from build123d import *

# Parameters (mm, degrees)
SKETCH1_R                             = 30
SKETCH1_R_2                           = 20
BOSS_EXTRUDE1_DEPTH                   = 40
TAP_DRILL_FOR_M8X1_25_TAP1_AT_2_COUNT = 2
TAP_DRILL_FOR_M8X1_25_TAP1_AT_2_PITCH = 40
TAP_DRILL_FOR_M8X1_25_TAP1_AT_3_COUNT = 2
TAP_DRILL_FOR_M8X1_25_TAP1_AT_3_PITCH = 50
TAP_DRILL_FOR_M8X1_25_TAP1_AT_4_COUNT = 2
TAP_DRILL_FOR_M8X1_25_TAP1_AT_4_PITCH = 30


with BuildPart() as part:
    # Sketch1 → Boss-Extrude1 (new, symmetric)
    with BuildSketch(Plane.XY):
        Circle(SKETCH1_R)
        Circle(SKETCH1_R_2, mode=Mode.SUBTRACT)
    extrude(amount=BOSS_EXTRUDE1_DEPTH, both=True)

    # Sketch12 → Tap Drill for M8x1.25 Tap1 (revolve, cut)
    with BuildSketch(Plane(origin=(-20, 15, 40), x_dir=(0, -1, 0), z_dir=(1, 0, 0))):
        Polygon((0, 0), (0, 22.042926105), (3.4, 20), (3.4, 0), align=None)
    tap_drill_for_m8x1_25_tap1 = revolve(axis=Axis((-20, 15, 46.35), (0, 0, -1)), mode=Mode.SUBTRACT)

    # Tap Drill for M8x1.25 Tap1 at 2: Tap Drill for M8x1.25 Tap1 ×2
    with Locations(*[(i * TAP_DRILL_FOR_M8X1_25_TAP1_AT_2_PITCH, 0, 0) for i in range(1, TAP_DRILL_FOR_M8X1_25_TAP1_AT_2_COUNT)]):
        add(tap_drill_for_m8x1_25_tap1, mode=Mode.SUBTRACT)

    # Tap Drill for M8x1.25 Tap1 at 3: Tap Drill for M8x1.25 Tap1 ×2
    with Locations(*[Vector(0.7999999999999999, -0.6000000000000001, 0) * (i * TAP_DRILL_FOR_M8X1_25_TAP1_AT_3_PITCH) for i in range(1, TAP_DRILL_FOR_M8X1_25_TAP1_AT_3_COUNT)]):
        add(tap_drill_for_m8x1_25_tap1, mode=Mode.SUBTRACT)

    # Tap Drill for M8x1.25 Tap1 at 4: Tap Drill for M8x1.25 Tap1 ×2
    with Locations(*[(0, -i * TAP_DRILL_FOR_M8X1_25_TAP1_AT_4_PITCH, 0) for i in range(1, TAP_DRILL_FOR_M8X1_25_TAP1_AT_4_COUNT)]):
        add(tap_drill_for_m8x1_25_tap1, mode=Mode.SUBTRACT)

    # Mirror1: Tap Drill for M8x1.25 Tap1 across plane
    add(tap_drill_for_m8x1_25_tap1.mirror(Plane.XY), mode=Mode.SUBTRACT)

    # Mirror1 copy 1 sketch → Mirror1 copy 1 (revolve, cut)
    with BuildSketch(Plane(origin=(20, 15, -40), x_dir=(0, -1, 0), z_dir=(1, 0, 0))):
        Polygon((0, 0), (0, -22.042926105), (3.4, -20), (3.4, 0), align=None)
    revolve(axis=Axis((20, 15, -46.35), (0, 0, -1)), mode=Mode.SUBTRACT)

    # Mirror1 copy 2 sketch → Mirror1 copy 2 (revolve, cut)
    with BuildSketch(Plane(origin=(20, -15, -40), x_dir=(0, -1, 0), z_dir=(1, 0, 0))):
        Polygon((0, 0), (0, -22.042926105), (3.4, -20), (3.4, 0), align=None)
    revolve(axis=Axis((20, -15, -46.35), (0, 0, -1)), mode=Mode.SUBTRACT)

    # Mirror1 copy 3 sketch → Mirror1 copy 3 (revolve, cut)
    with BuildSketch(Plane(origin=(-20, -15, -40), x_dir=(0, -1, 0), z_dir=(1, 0, 0))):
        Polygon((0, 0), (0, -22.042926105), (3.4, -20), (3.4, 0), align=None)
    revolve(axis=Axis((-20, -15, -46.35), (0, 0, -1)), mode=Mode.SUBTRACT)


solid = part.part
Model file for the job. Use its own axes, mm. A direction names the side the tool comes from. Round coordinates to 2 decimals unless told otherwise and drop trailing zeros. Loops run counter-clockwise (first coordinate to the right, second up) from the corner with the lowest first, then second, coordinate; pieces in that order, holes last. Notation, with made-up numbers: (7, -19.75) -> (37, -19.75) arc R22 ccw to (37, -12.75) -> close; hole circle Ø4 at (7, 18). An arc over 180 degrees is marked (long way). Answer as CSV lines item,"result". Start each with the question number.
1) Slice it at B-B (y = -6). List the corners of the cut face in (x, z).
2) Tool access for faces 1 (the face through (23.32, -14.26, -30.14)), 2 (the face through (-16.68, -14.26, 30.14)): list every direction of +Z, -Z, +X, -X, +Y, -Y with a clear straight run to the whole face (end or side of a thin tool).
3) Slice it at D-D (z = 2). List the corners of the cut face in (x, y).
4) Slice it at A-A (x = 0). List the corners of the cut face in (y, z), plus the area to 3 significant figures.
5) Mould opens along Y. For faces 3 (the face through (-4.336, -19.524, -0.56)), 4 (the face through (20, -6, 40)), 5 (the face through (-29.97, 1.32, 0.56)), 6 (the face through (-16.68, 15.74, -30.14)) say: +Y half, -Y half, draft (parallel to the pull), parting line (faces both ways), or undercut.
6) Slice it at C-C (z = -32). List the corners of the cut face in (x, y), plus the area to 3 significant figures.
7) Pin check, flat tips, straight feed: P1, Ø1, axis at y = -16, z = 4.5, coming from the -X side; P2, Ø8, axis at x = -12.5, z = 15.5, coming from the -Y side; P3, Ø8, axis at x = -12.5, z = -16, coming from the +Y side. Stop position of each tip, or through.
8) Probe line 1 along X through (y, z) = (-15, 29); line 2 along X through (y, z) = (-16, 20.5); line 3 along Y through (x, z) = (-5, -31.5). List the from-to ranges inside material, lowest first.
Filled in:
1,outline,"(-29.39, -40) -> (-19.08, -40) -> (-19.08, 40) -> (-29.39, 40) -> close; (19.08, -40) -> (29.39, -40) -> (29.39, 40) -> (19.08, 40) -> close"
2,face 1,"-Z"
2,face 2,"+Z"
3,outline,"circle Ø60 at (0, 0); hole circle Ø40 at (0, 0)"
4,outline,"(-30, -40) -> (-20, -40) -> (-20, 40) -> (-30, 40) -> close; (20, -40) -> (30, -40) -> (30, 40) -> (20, 40) -> close"
4,area,"1,600 mm2"
5,face 3,"undercut"
5,face 4,"draft"
5,face 5,"parting line"
5,face 6,"undercut"
6,outline,"circle Ø60 at (0, 0); hole circle Ø6.8 at (-20, -15); hole circle Ø6.8 at (-20, 15); hole circle Ø40 at (0, 0); hole circle Ø6.8 at (20, -15); hole circle Ø6.8 at (20, 15)"
6,area,"1,430 mm2"
7,P1,"stops at x = -25.69"
7,P2,"stops at y = -28.77"
7,P3,"stops at y = 28.77"
8,line 1,"x = -25.98 to -23.4, -16.6 to -13.23, 13.23 to 16.6, 23.4 to 25.98"
8,line 2,"x = -25.38 to -23.25, -16.75 to -12, 12 to 16.75, 23.25 to 25.38"
8,line 3,"y = -29.58 to -19.36, 19.36 to 29.58"
